Model file for the job. Use its own axes, mm. Face numbers are marked on the shaded views. A direction names the side the tool comes from. Give positions to 0.01 mm unless a question says otherwise; leave off trailing zeros. Loops run counter-clockwise (first coordinate to the right, second up) from the corner with the lowest first, then second, coordinate; pieces in that order, holes last. Notation, with made-up numbers: (-36, -40) - (-15, -40) arc R14 ccw to (-15, -25) - close; hole circle Ø3 at (56.25, 6.25). An arc over 180 degrees is marked (long way). Answer as CSV lines item,"result". Start each with the question number.
Item 1: Saw through at B-B on z = 33.5. Give the cut face in (x, y), plus the area to 3 significant figures.
Item 2: Tool access for the marked faces 5 and 6: list every direction of +Z, -Z, +X, -X, +Y, -Y with a clear straight run to the whole face (end or side of a thin tool).
Item 3: Pull direction X, two halves, no side cores. Call the marked faces 1, 2, 3 and 4: pulls with the +X half, pulls with the -X half, needs draft (parallel to the pull), parting line crosses it, or undercut.
Item 4: Saw through at D-D on x = -14.5. Give the cut face in (y, z), plus the area to 3 significant figures.
Item 5: Pin check, flat tips, straight feed: pin 1 (2.5 mm diameter, centred on y = 22.5, z = 16.9, fed in from +X); pin 2 (10.5 mm diameter, centred on x = -24.5, z = 29, fed in from +Y). Stop position of each tip, or through.
Item 6: Drill centre lines: L1, parallel to X at y = 16, z = 29.5; L2, parallel to Y at x = -4, z = 17; L3, parallel to Y at x = -13, z = 24.5. Where is each one in solid material? Low to high. Write a range as from..to.
Item 7: Saw through at C-C on y = 22.5. Give the cut face in (x, z).
Item 8: Saw through at A-A on y = 12.5. Give the cut face in (x, z), plus the area to 3 significant figures.
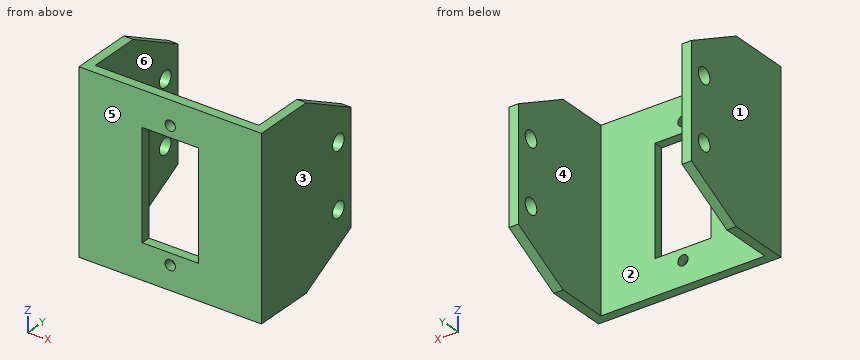
from build123d import *

# Parameters (mm, degrees)
SKETCH_2_R          = 1.1
SKETCH_2_W          = 12
SKETCH_2_H          = 23
EXTRUDE_2_DEPTH     = 2
SKETCH_4_W          = 2
SKETCH_4_H          = 38
EXTRUDE_3_DEPTH     = 24.2
SKETCH_5_W          = 2
SKETCH_5_H          = 38
EXTRUDE_4_DEPTH     = 24.2
SKETCH_6_R          = 1.7
CUT_EXTRUDE_1_DEPTH = 50
CUT_EXTRUDE_2_DEPTH = 39


with BuildPart() as part:
    # 草图2 → 凸台-拉伸2 (new body)
    with BuildSketch(Plane(origin=(0, 0, 0), x_dir=(1, 0, 0), z_dir=(0, 1, 0))):
        Polygon((-39.22677438, -4.600854345), (-4.22677438, -4.600854345), (-2.22677438, -4.600854345), (-2.22677438, -42.600854345), (-4.22677438, -42.600854345), (-39.22677438, -42.600854345), (-41.22677438, -42.600854345), (-41.22677438, -4.600854345), align=None)
        with Locations(Location((-21.72677438, -9.700854345, 0), (0, 0, 270))):
            Circle(SKETCH_2_R, mode=Mode.SUBTRACT)
        with Locations(Location((-21.72677438, -37.500854345, 0), (0, 0, 90))):
            Circle(SKETCH_2_R, mode=Mode.SUBTRACT)
        with Locations((-21.72677438, -23.600854345)):
            Rectangle(SKETCH_2_W, SKETCH_2_H, mode=Mode.SUBTRACT)
    extrude(amount=EXTRUDE_2_DEPTH)

    # 草图4 → 凸台-拉伸3 (add)
    with BuildSketch(Plane(origin=(0, 2, 0), x_dir=(1, 0, 0), z_dir=(0, 1, 0))):
        with Locations((-40.22677438, -23.600854345)):
            Rectangle(SKETCH_4_W, SKETCH_4_H)
    extrude(amount=EXTRUDE_3_DEPTH)

    # 草图5 → 凸台-拉伸4 (add)
    with BuildSketch(Plane(origin=(0, 2, 0), x_dir=(1, 0, 0), z_dir=(0, 1, 0))):
        with Locations((-3.22677438, -23.600854345)):
            Rectangle(SKETCH_5_W, SKETCH_5_H)
    extrude(amount=EXTRUDE_4_DEPTH)

    # 草图6 → 切除-拉伸1 (cut)
    with BuildSketch(Plane(origin=(-2.22677438, 0, 0), x_dir=(0, 0, -1), z_dir=(1, 0, 0))):
        with Locations((-30.300854345, 22.5)):
            Circle(SKETCH_6_R)
        with Locations((-16.900854345, 22.5)):
            Circle(SKETCH_6_R)
    extrude(amount=-CUT_EXTRUDE_1_DEPTH, mode=Mode.SUBTRACT)

    # 草图7 → 切除-拉伸2 (cut)
    with BuildSketch(Plane(origin=(-2.22677438, 0, 0), x_dir=(0, 0, -1), z_dir=(1, 0, 0))):
        Polygon((-35.600854345, 26.2), (-42.600854345, 13.1), (-42.600854345, 26.2), align=None)
        Polygon((-11.600854345, 26.2), (-4.600854345, 13.1), (-4.600854345, 26.2), align=None)
    extrude(amount=-CUT_EXTRUDE_2_DEPTH, mode=Mode.SUBTRACT)


solid = part.part
Responses:
1,outline,"(-41.23, 0) - (-27.73, 0) - (-27.73, 2) - (-39.23, 2) - (-39.23, 26.2) - (-41.23, 26.2) - close; (-15.73, 0) - (-2.23, 0) - (-2.23, 26.2) - (-4.23, 26.2) - (-4.23, 2) - (-15.73, 2) - close"
1,area,"151 mm2"
2,face 5,"+Z, -Z, +X, -X, -Y"
2,face 6,"+Z, -Z, +Y"
3,face 1,"pulls with the -X half"
3,face 2,"undercut"
3,face 3,"pulls with the +X half"
3,face 4,"undercut"
4,outline,"(0, 4.6) - (2, 4.6) - (2, 42.6) - (0, 42.6) - close"
4,area,"76.0 mm2"
5,pin 1,"through"
5,pin 2,"y = 2"
6,L1,"-41.23..-39.23, -4.23..-2.23"
6,L2,"0..20.8, 24.2..26.2"
6,L3,"0..2"
7,outline,"(-41.23, 9.62) - (-39.23, 9.62) - (-39.23, 15.2) - (-41.23, 15.2) - close; (-41.23, 18.6) - (-39.23, 18.6) - (-39.23, 28.6) - (-41.23, 28.6) - close; (-41.23, 32) - (-39.23, 32) - (-39.23, 37.58) - (-41.23, 37.58) - close; (-4.23, 9.62) - (-2.23, 9.62) - (-2.23, 15.2) - (-4.23, 15.2) - close; (-4.23, 18.6) - (-2.23, 18.6) - (-2.23, 28.6) - (-4.23, 28.6) - close; (-4.23, 32) - (-2.23, 32) - (-2.23, 37.58) - (-4.23, 37.58) - close"
8,outline,"(-41.23, 4.6) - (-39.23, 4.6) - (-39.23, 42.6) - (-41.23, 42.6) - close; (-4.23, 4.6) - (-2.23, 4.6) - (-2.23, 42.6) - (-4.23, 42.6) - close"
8,area,"152 mm2"
